The drawing under review shows one solid part. Ordinate dimensions are in mm from its lowest x, y, z. A direction names the side the tool comes from. Coordinates: 2 decimals unless noted, no trailing zeros. Write each loop counter-clockwise with the first axis right and the second up, starting at its lowest first coordinate (ties: lowest second). Pieces come first, ordered by that corner, then holes.
Q1. Insertion check: pin 1 (12 mm diameter, centred on y = 35, z = 84, fed in from -X); pin 2 (4 mm diameter, centred on y = 12, z = 31, fed in from +X); pin 3 (1.5 mm diameter, centred on x = 11, y = 41.5, fed in from +Z). Each pin has a flat end and moves straight along its axis. Give the tip position at first contact, or say it passes through.
Q2. Take a section at B-B (y = 47.5). Give the boundary of the cut face in (x, z), and give its area (3 significant figures).
Q3. Take a section at A-A (x = 65). Give the boundary of the cut face in (y, z).
Q4. Take a section at D-D (x = 56.5). Give the boundary of the cut face in (y, z).
Q5. For probe 1 along Z at (x, y) = (63, 3.5); probe 2 along Y at (x, z) = (65, 6); probe 3 along Y at (x, z) = (16, 96), list the stretches that pass through material, from the lowest coordinate up.
Q6. Machinability: for the marked faces 1, 2 and 3, which of the approach directions +Z, -Z, +X, -X, +Y, -Y give a long, thin tool a straight path to every point of the face, cutting with its end or side? Answer none if there is none.
Q7. Mouldability with a two-part tool opening along Z and no side actions: class the marked faces 4, 5, 6 and 7 as pulls with the +Z half, pulls with the -Z half, needs draft (parallel to the pull), parting line crosses it, or undercut.
Q8. Take a section at C-C (z = 10). Give the boundary of the cut face in (x, y).
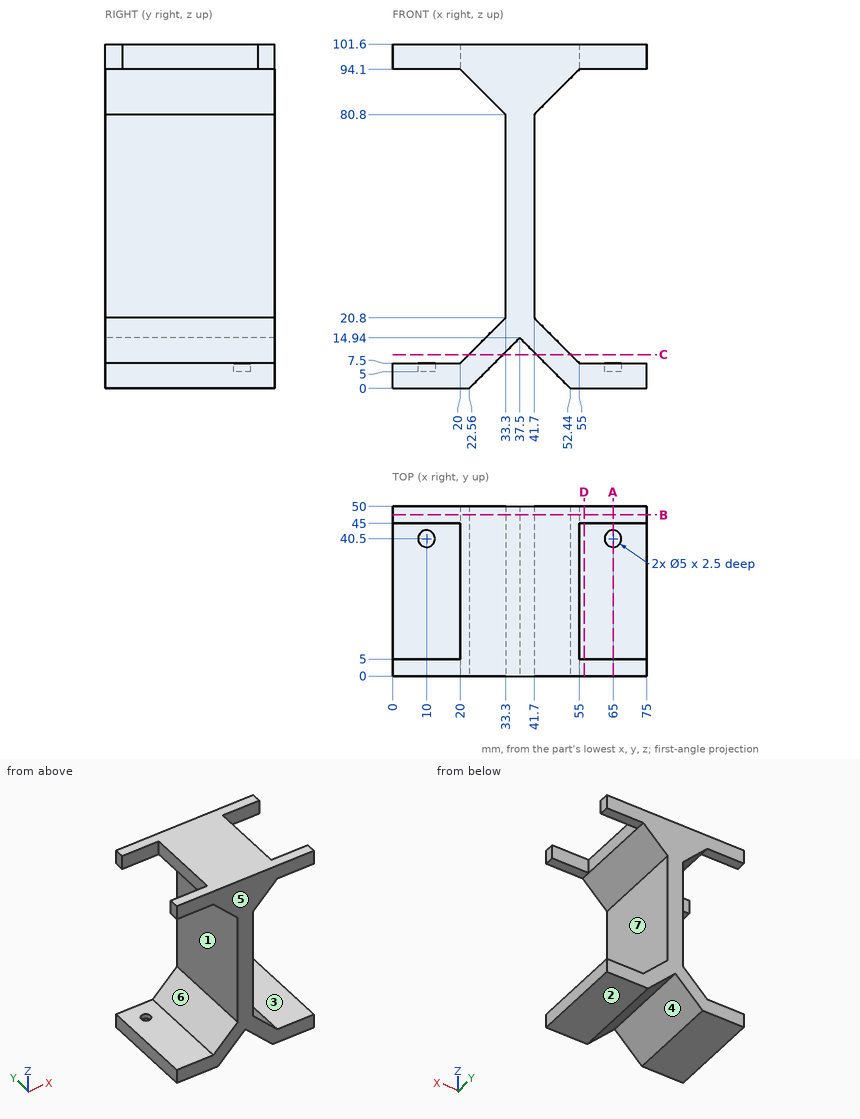
Response:
1. pin 1: stops at x = 24.1
1. pin 2: stops at x = 41.7
1. pin 3: stops at z = 5
2. outline: (0, 0) - (22.56, 0) - (37.5, 14.94) - (52.44, 0) - (75, 0) - (75, 7.5) - (55, 7.5) - (41.7, 20.8) - (41.7, 80.8) - (55, 94.1) - (75, 94.1) - (75, 101.6) - (0, 101.6) - (0, 94.1) - (20, 94.1) - (33.3, 80.8) - (33.3, 20.8) - (20, 7.5) - (0, 7.5) - close
2. area: 1,980 mm2
3. outline: (0, 0) - (50, 0) - (50, 7.5) - (43, 7.5) - (43, 5) - (38, 5) - (38, 7.5) - (0, 7.5) - close; (0, 94.1) - (5, 94.1) - (5, 101.6) - (0, 101.6) - close; (45, 94.1) - (50, 94.1) - (50, 101.6) - (45, 101.6) - close
4. outline: (0, 0) - (50, 0) - (50, 7.5) - (0, 7.5) - close; (0, 94.1) - (5, 94.1) - (5, 101.6) - (0, 101.6) - close; (45, 94.1) - (50, 94.1) - (50, 101.6) - (45, 101.6) - close
5. probe 1: z = 0 to 7.5, 94.1 to 101.6
5. probe 2: y = 0 to 38, 43 to 50
5. probe 3: y = 0 to 5, 45 to 50
6. face 1: -X, +Y, -Y
6. face 2: -Z, +X, -X, +Y, -Y
6. face 3: +X, +Y, -Y
7. face 4: pulls with the -Z half
7. face 5: needs draft
7. face 6: undercut
7. face 7: undercut
8. outline: (22.5, 0) - (32.56, 0) - (32.56, 50) - (22.5, 50) - close; (42.44, 0) - (52.5, 0) - (52.5, 50) - (42.44, 50) - close
